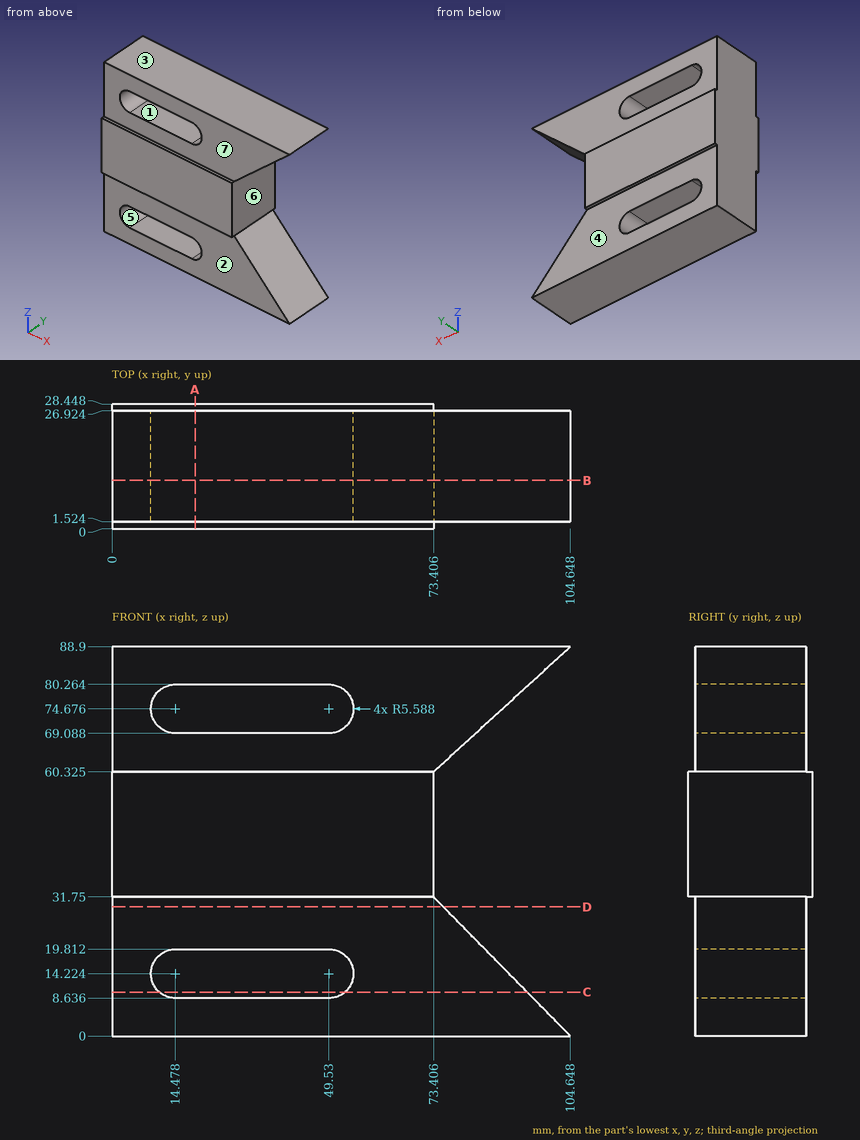
Geometry check sheet. Reference: drawing and pictorial views, mm from the part's lowest x, y, z. A direction names the side the tool comes from. Round coordinates to 2 decimals unless told otherwise and drop trailing zeros. Order: outer loops, then holes, each group sorted by start corner. A loop starts at its lowest first (then second) coordinate and runs counter-clockwise, first axis right, second up. Notation, with made-up numbers: (38.25, -20) -> (74.25, -20) arc R30 cw to (74.25, 15) -> close; hole circle Ø9 at (67, -6). An arc over 180 degrees is marked (long way). One line per item, written item: value. Start each with the question number.
Q1. Cross-section at D-D (z = 29.5). Record the boundary of the cut face in (x, y), and give its area (3 significant figures).
Q2. Set-up check for the marked faces 4, 5, 6 and 7: record each of +Z, -Z, +X, -X, +Y, -Y from which the full face is reachable in a straight line by a thin tool's end or side.
Q3. Gauge pin test, flat ends, axial feed: pin 1 Ø5 at (x, y) = (18, 13.5) entering from -Z; pin 2 Ø8 at (x, z) = (78, 9) entering from +Y; pin 3 Ø1.7 at (x, y) = (29, 0.5) entering from -Z; pin 4 Ø8 at (y, z) = (6, 27.5) entering from +X. Record the tip position at first contact, or that the pin passes through.
Q4. Cross-section at B-B (y = 11). Record the boundary of the cut face in (x, z) (3 decimals), and give its area (3 significant figures).
Q5. Cross-section at C-C (z = 10). Record the boundary of the cut face in (x, y).
Q6. Thickness scan on line 1 (Z direction, x = 37.5, y = 26); line 2 (Z direction, x = 52, y = 10); line 3 (Y direction, x = 5, z = 29). Record the ranges inside material, lowest first.
Q7. Mould release check, pull along Z, two halves, no side actions. Record for the marked faces 1, 2 and 3: pulls with the +Z half, pulls with the -Z half, needs draft (parallel to the pull), parting line crosses it, or undercut.
Q8. Cross-section at A-A (x = 19). Record the boundary of the cut face in (y, z) (3 decimals), and give its area (3 significant figures).
Completed:
1. outline: (0, 1.52) -> (75.62, 1.52) -> (75.62, 26.92) -> (0, 26.92) -> close
1. area: 1,920 mm²
2. face 4: -Z, +X, -X, +Y
2. face 5: +Y, -Y
2. face 6: +X, +Y, -Y
2. face 7: +Z, +X, -X, -Y
3. pin 1: stops at z = 0
3. pin 2: stops at y = 26.92
3. pin 3: stops at z = 31.75
3. pin 4: stops at x = 81.52
4. outline: (0, 0) -> (104.648, 0) -> (73.406, 31.75) -> (73.406, 60.325) -> (104.648, 88.9) -> (0, 88.9) -> close; hole (14.478, 8.636) -> (49.53, 8.636) arc R5.588 ccw to (49.53, 19.812) -> (14.478, 19.812) arc R5.588 ccw to start; hole (14.478, 69.088) -> (49.53, 69.088) arc R5.588 ccw to (49.53, 80.264) -> (14.478, 80.264) arc R5.588 ccw to start
4. area: 6,490 mm²
5. outline: (0, 1.52) -> (10.82, 1.52) -> (10.82, 26.92) -> (0, 26.92) -> close; (53.19, 1.52) -> (94.81, 1.52) -> (94.81, 26.92) -> (53.19, 26.92) -> close
6. line 1: z = 0 to 8.64, 19.81 to 69.09, 80.26 to 88.9
6. line 2: z = 0 to 9.21, 19.24 to 69.66, 79.69 to 88.9
6. line 3: y = 1.52 to 26.92
7. face 1: undercut
7. face 2: needs draft
7. face 3: pulls with the +Z half
8. outline: (0, 31.75) -> (1.524, 31.75) -> (1.524, 19.812) -> (26.924, 19.812) -> (26.924, 31.75) -> (28.448, 31.75) -> (28.448, 60.325) -> (26.924, 60.325) -> (26.924, 69.088) -> (1.524, 69.088) -> (1.524, 60.325) -> (0, 60.325) -> close; (1.524, 0) -> (26.924, 0) -> (26.924, 8.636) -> (1.524, 8.636) -> close; (1.524, 80.264) -> (26.924, 80.264) -> (26.924, 88.9) -> (1.524, 88.9) -> close
8. area: 1,780 mm²
